```python
from build123d import *

# Parameters (mm, degrees)
BOSS_EXTRUDE1_DEPTH = 16
FILLET1_R           = 1
FILLET2_R           = 3
FILLET3_R           = 3
FILLET4_R           = 3
SKETCH2_W           = 7.425804379
SKETCH2_H           = 16
CUT_EXTRUDE1_DEPTH  = 13
FILLET5_R           = 3
SKETCH3_W           = 17.675238391
SKETCH3_H           = 28.7828695
CUT_EXTRUDE2_DEPTH  = 33
FILLET6_R           = 1
SKETCH4_W           = 6.794443954
SKETCH4_H           = 18.076730961
CUT_EXTRUDE3_DEPTH  = 33


with BuildPart() as part:
    # Sketch1 → Boss-Extrude1 (new body)
    with BuildSketch(Plane.XY):
        Polygon((0, 0), (21.560913706, 0), (21.560913706, 30), (16.560913706, 30), (16.560913706, 5), (0, 5), align=None)
    extrude(amount=BOSS_EXTRUDE1_DEPTH)

    # Fillet1
    fillet1_edges = [part.edges().sort_by_distance(p)[0] for p in [
        (21.560913706, 30, 8),
        (0, 0, 8),
        (21.560913706, 15, 16),
        (21.560913706, 15, 0),
        (10.780456853, 0, 0),
        (10.780456853, 0, 16),
    ]]
    fillet(fillet1_edges, radius=FILLET1_R)

    # Fillet2
    # the kernel refuses this fillet: 3 mm, written as the material it takes off along each edge
    with BuildSketch(Plane(origin=(18.560913706, 3, 16), x_dir=(0, -1, 0), z_dir=(-1, 0, 0))) as fillet2_piece_1:
        with BuildLine():
            CenterArc((2, -1), 1, 0, 90)
            Line((3, -1), (3, 0))
            Line((3, 0), (2, 0))
        make_face()
    revolve(axis=Axis((18.560913706, 3, 16), (0, 0, 1)), revolution_arc=90, mode=Mode.SUBTRACT)
    with BuildSketch(Plane(origin=(18.560913706, 3, 0), x_dir=(1, 0, 0), z_dir=(0, 1, 0))) as fillet2_piece_2:
        with BuildLine():
            CenterArc((2, -1), 1, 0, 90)
            Line((3, -1), (3, 0))
            Line((3, 0), (2, 0))
        make_face()
    revolve(axis=Axis((18.560913706, 3, 0), (0, 0, -1)), revolution_arc=90, mode=Mode.SUBTRACT)
    with BuildSketch(Plane(origin=(21.560913706, 0, 0), x_dir=(-1, 0, 0), z_dir=(0, 0, 1))) as fillet2_piece_3:
        with BuildLine():
            CenterArc((FILLET2_R, -FILLET2_R), FILLET2_R, 90, 90)
            Line((0, -FILLET2_R), (0, 0))
            Line((0, 0), (FILLET2_R, 0))
        make_face()
    extrude(amount=16, mode=Mode.SUBTRACT)

    # Fillet3
    fillet3_edges = [part.edges().sort_by_distance(p)[0] for p in [
        (16.560913706, 5, 8),
    ]]
    fillet(fillet3_edges, radius=FILLET3_R)

    # Fillet4
    fillet4_edges = [part.edges().sort_by_distance(p)[0] for p in [
        (0, 5, 8),
        (16.560913706, 30, 8),
    ]]
    fillet(fillet4_edges, radius=FILLET4_R)

    # Sketch2 → Cut-Extrude1 (cut)
    with BuildSketch(Plane.XZ):
        with Locations((3.71290219, 8)):
            Rectangle(SKETCH2_W, SKETCH2_H)
    extrude(amount=-CUT_EXTRUDE1_DEPTH, mode=Mode.SUBTRACT)

    # Fillet5
    fillet5_edges = [part.edges().sort_by_distance(p)[0] for p in [
        (7.425804379, 5, 8),
    ]]
    fillet(fillet5_edges, radius=FILLET5_R)

    # Sketch3 → Cut-Extrude2 (cut)
    with BuildSketch(Plane(origin=(0, 0, 0), x_dir=(-1, 0, 0), z_dir=(0, 0, -1))):
        with Locations((-10.361055803, 16.45457074)):
            Rectangle(SKETCH3_W, SKETCH3_H)
    extrude(amount=-CUT_EXTRUDE2_DEPTH, mode=Mode.SUBTRACT)

    # Fillet6
    fillet6_edges = [part.edges().sort_by_distance(p)[0] for p in [
        (19.198674998, 2.06313599, 8),
    ]]
    fillet(fillet6_edges, radius=FILLET6_R)

    # Sketch4 → Cut-Extrude3 (cut)
    with BuildSketch(Plane(origin=(0, 2.06313599, 0), x_dir=(1, 0, 0), z_dir=(0, 1, 0))):
        with Locations((10.074463298, -8.207535366)):
            Rectangle(SKETCH4_W, SKETCH4_H)
    extrude(amount=-CUT_EXTRUDE3_DEPTH, mode=Mode.SUBTRACT)


solid = part.part
```
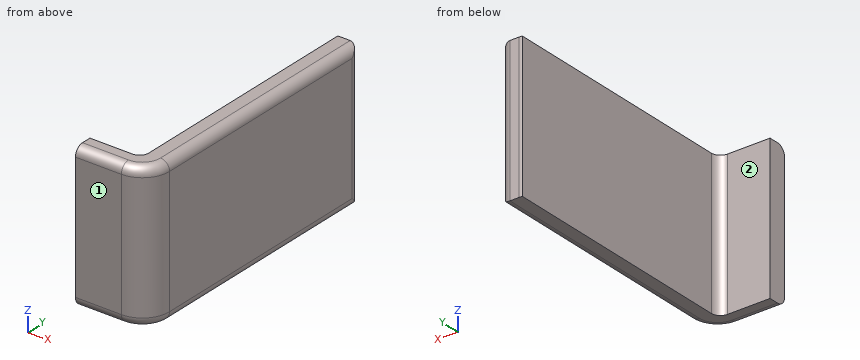
Geometry: final body of the model. Coordinates: model frame, mm. Face numbers are marked on the shaded views. A direction names the side the tool comes from. Round coordinates to 2 decimals unless told otherwise and drop trailing zeros. Write each loop counter-clockwise with the first axis right and the second up, starting at its lowest first coordinate (ties: lowest second). Pieces come first, ordered by that corner, then holes. Notation, with made-up numbers: (58.25, 32.5) -> (72.25, 32.5) arc R20 cw to (72.25, 54.5) -> close; hole circle Ø11 at (4, 41). An arc over 180 degrees is marked (long way). Use CSV: the item, a comma, the result in double quotes. Start each with the question number.
Q1. Section C-C (x = 16.25). Return loops of the section in (y, z), plus the area to 3 significant figures.
Q2. Section B-B (y = 5.75). Return loops of the section in (x, z), plus the area to 3 significant figures.
Q3. Reachability of the marked faces 1 and 2 from +Z, -Z, +X, -X, +Y, -Y: full face, straight path, thin tool, end or side. Return the list, or none.
Q4. First-contact query: pin 1 Ø5 at (y, z) = (16.5, 4) entering from -X; pin 2 Ø2 at (x, z) = (18, 9) entering from +Y. Flat tips, straight axial feed; report the tip coordinate or a pass-through.
Q5. Line query: L1, parallel to X at y = 10.25, z = 7.25; L2, parallel to Y at x = 14.75, z = 3.25; L3, parallel to Y at x = 19.25, z = 5. Output: solid intervals per line, ascending.
Q6. Section A-A (z = 12.5). Return loops of the section in (x, y), plus the area to 3 significant figures.
Result sheet:
1,outline,"(0, 1) arc R1 ccw to (1, 0) -> (2.06, 0) -> (2.06, 16) -> (1, 16) arc R1 ccw to (0, 15) -> close"
1,area,"32.6 mm²"
2,outline,"(19.2, 0) -> (20.56, 0) arc R1 ccw to (21.56, 1) -> (21.56, 15) arc R1 ccw to (20.56, 16) -> (19.2, 16) -> close"
2,area,"37.4 mm²"
3,face 1,"+Z, -Z, +X, -X, -Y"
3,face 2,"+Z, -Z, -X, +Y"
4,pin 1,"x = 19.2"
4,pin 2,"y = 2.46"
5,L1,"19.2 to 21.56"
5,L2,"0 to 2.06"
5,L3,"0.08 to 29.98"
6,outline,"(13.47, 0) -> (18.56, 0) arc R3 ccw to (21.56, 3) -> (21.56, 29) arc R1 ccw to (20.56, 30) -> (19.56, 30) arc R3 ccw to (19.2, 29.98) -> (19.2, 3.06) arc R1 cw to (18.2, 2.06) -> (13.47, 2.06) -> close"
6,area,"80.7 mm²"
